from build123d import *

# Parameters (mm, degrees)
SKETCH1_R           = 36.25
SKETCH1_R_2         = 26.25
BOSS_EXTRUDE1_DEPTH = 16
BOSS_EXTRUDE2_START = 12
SKETCH2_R           = 36.25
SKETCH2_R_2         = 14
BOSS_EXTRUDE2_DEPTH = 12
SKETCH4_W           = 15
SKETCH4_H           = 30
CUT_EXTRUDE1_DEPTH  = 10
SKETCH5_R           = 22.5
CUT_EXTRUDE2_DEPTH  = 10
SKETCH7_R           = 2.5
CUT_EXTRUDE3_DEPTH  = 59.413397436


with BuildPart() as part:
    # Sketch1 → Boss-Extrude1 (new body)
    with BuildSketch(Plane.XY):
        Circle(SKETCH1_R)
        Circle(SKETCH1_R_2, mode=Mode.SUBTRACT)
    extrude(amount=BOSS_EXTRUDE1_DEPTH)

    # Sketch2 → Boss-Extrude2 (add)
    with BuildSketch(Plane(origin=(0, 0, 0), x_dir=(-1, 0, 0), z_dir=(0, 0, -1)).offset(BOSS_EXTRUDE2_START)):
        Circle(SKETCH2_R)
        Circle(SKETCH2_R_2, mode=Mode.SUBTRACT)
    extrude(amount=-BOSS_EXTRUDE2_DEPTH)

    # Sketch4 → Cut-Extrude1 (cut)
    with BuildSketch(Plane(origin=(0, 0, -12), x_dir=(-1, 0, 0), z_dir=(0, 0, -1))):
        with Locations((0, 23)):
            Rectangle(SKETCH4_W, SKETCH4_H)
    extrude(amount=-CUT_EXTRUDE1_DEPTH, mode=Mode.SUBTRACT)

    # Sketch5 → Cut-Extrude2 (cut)
    with BuildSketch(Plane(origin=(0, 0, -12), x_dir=(-1, 0, 0), z_dir=(0, 0, -1))):
        Circle(SKETCH5_R)
    extrude(amount=-CUT_EXTRUDE2_DEPTH, mode=Mode.SUBTRACT)

    # Sketch7 → Cut-Extrude3 (cut, through all)
    with BuildSketch(Plane(origin=(0, 0, -12), x_dir=(-1, 0, 0), z_dir=(0, 0, -1))):
        with Locations((-25.980762114, 15)):
            Circle(SKETCH7_R)
        with Locations((25.980762114, 15)):
            Circle(SKETCH7_R)
        with Locations((0, -30)):
            Circle(SKETCH7_R)
    extrude(amount=-CUT_EXTRUDE3_DEPTH, mode=Mode.SUBTRACT)


solid = part.part
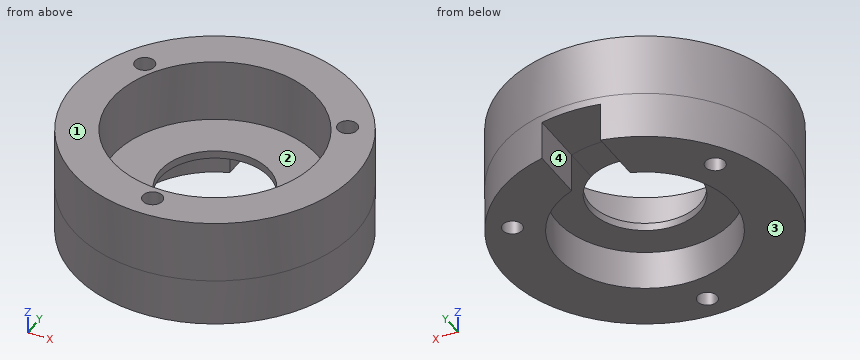
The listing builds one solid part. Answer for the finished solid, in the listing's coordinates (mm). Face numbers are marked on the shaded views. A direction names the side the tool comes from. Give positions to 0.01 mm unless a question says otherwise; leave off trailing zeros. Loops run counter-clockwise (first coordinate to the right, second up) from the corner with the lowest first, then second, coordinate; pieces in that order, holes last. Notation, with made-up numbers: (2.5, 63.25) - (45.5, 63.25) arc R14 cw to (45.5, 87.25) - close; hole circle Ø8 at (88.5, 81.25). An arc over 180 degrees is marked (long way). Use one line per item in the form item = value.
1. Section A-A on x = 0 is taken. Give the vertices of the cut face in (y, z), then the cut area to 4 significant figures.
Calculated:
outline = (-36.25, -12) - (-32.5, -12) - (-32.5, 16) - (-36.25, 16) - close; (-27.5, -12) - (-22.5, -12) - (-22.5, -2) - (-14, -2) - (-14, 0) - (-26.25, 0) - (-26.25, 16) - (-27.5, 16) - close; (14, -2) - (36.25, -2) - (36.25, 16) - (26.25, 16) - (26.25, 0) - (14, 0) - close
area = 406.5 mm^2
2. Find the intervals of material crossed by line 1 along Y through (x, z) = (0, 3.5); line 2 along Y through (x, z) = (0, -1.45); line 3 along X through (y, z) = (0, -1.3), in increasing order. Write a range as [from, to].
Calculated:
line_1 = [-36.25, -32.5], [-27.5, -26.25], [26.25, 36.25]
line_2 = [-36.25, -32.5], [-27.5, -14], [14, 36.25]
line_3 = [-36.25, -14], [14, 36.25]
3. Given pin 1 Ø8 at (y, z) = (27, -5.5) entering from +X; pin 2 Ø22 at (x, y) = (0.5, 2.5) entering from -Z; pin 3 Ø10 at (x, y) = (16.5, 11.5) entering from +Z; pin 4 Ø4.5 at (x, y) = (-0.5, 30.5) entering from -Z, each flat-ended and moving along its own axis, determine where each tip first touches the part or whether it passes through.
Calculated:
pin_1 = 28.02
pin_2 = through
pin_3 = 0
pin_4 = -2
4. The mould has two halves that part along X. Classify the marked faces 3 and 4: pulls with the +X half, pulls with the -X half, needs draft (parallel to the pull), parting line crosses it, or undercut.
Calculated:
face_3 = needs draft
face_4 = undercut
5. Section D-D on z = -7.75 is taken. Give the vertices of the cut face in (x, y), then the cut area to 3 significant figures.
Calculated:
outline = (-7.5, 21.21) - (-7.5, 35.47) arc R36.25 ccw (long way) to (7.5, 35.47) - (7.5, 21.21) arc R22.5 cw (long way) to start; hole circle Ø5 at (-25.98, 15); hole circle Ø5 at (0, -30); hole circle Ø5 at (25.98, 15)
area = 2,270 mm^2
6. Section C-C on x = -13 is taken. Give the vertices of the cut face in (y, z).
Calculated:
outline = (-33.84, -12) - (-18.36, -12) - (-18.36, -2) - (-5.2, -2) - (-5.2, 0) - (-22.8, 0) - (-22.8, 16) - (-33.84, 16) - close; (5.2, -2) - (18.36, -2) - (18.36, -12) - (33.84, -12) - (33.84, 16) - (22.8, 16) - (22.8, 0) - (5.2, 0) - close
7. Section B-B on z = 13.25 is taken. Give the vertices of the cut face in (x, y).
Calculated:
outline = circle Ø72.5 at (0, 0); hole circle Ø5 at (-25.98, 15); hole circle Ø52.5 at (0, 0); hole circle Ø5 at (0, -30); hole circle Ø5 at (25.98, 15)
8. Which of the six approach directions +Z, -Z, +X, -X, +Y, -Y give full straight-line access (tool end or side, diameter ignored) to the marked faces 1 and 2?
Calculated:
face_1 = +Z, +X, -X, +Y, -Y
face_2 = +Z
